Geometry check sheet. Reference: the model listing, model coordinates, mm. A direction names the side the tool comes from. Give positions to 0.01 mm unless a question says otherwise; leave off trailing zeros. Order: outer loops, then holes, each group sorted by start corner. A loop starts at its lowest first (then second) coordinate and runs counter-clockwise, first axis right, second up. Notation, with made-up numbers: M 77,68 L 96,68 A21 ccw 96,97 Z; hole C 79.5,-36 d7. An arc over 180 degrees is marked long. Use CSV: the item, a comma, the result in double quotes. Start each with the question number.
from build123d import *

# Parameters (mm, degrees)
SKETCH1_R                        = 8
BOSS_EXTRUDE1_DEPTH              = 21.88
BOSS_EXTRUDE2_DEPTH              = 26.5
SKETCH3_R                        = 2.835
BOSS_EXTRUDE3_DEPTH              = 2
BOSS_EXTRUDE4_DEPTH              = 10
F_2_05_2_05_DIAMETER_HOLE1_D     = 2.05
F_2_05_2_05_DIAMETER_HOLE1_DEPTH = 3
F_2_05_2_05_DIAMETER_HOLE1_TIP   = 0.615882135


with BuildPart() as part:
    # Sketch1 → Boss-Extrude1 (new body)
    with BuildSketch(Plane.XY):
        Circle(SKETCH1_R)
    extrude(amount=BOSS_EXTRUDE1_DEPTH)

    # Sketch2 → Boss-Extrude2 (add)
    with BuildSketch(Plane.XY.offset(21.88)):
        with BuildLine():
            Line((5.634523633, 5.0703593), (6.054375133, -4.560804945))
            ThreePointArc((6.054375133, -4.560804945), (0.33012154, -7.572807918), (-5.634523633, -5.0703593))
            Line((-5.634523633, -5.0703593), (-6.054375133, 4.560804945))
            ThreePointArc((-6.054375133, 4.560804945), (-0.33012154, 7.572807918), (5.634523633, 5.0703593))
        make_face()
    extrude(amount=BOSS_EXTRUDE2_DEPTH)

    # Sketch3 → Boss-Extrude3 (add)
    with BuildSketch(Plane(origin=(0, 0, 0), x_dir=(-1, 0, 0), z_dir=(0, 0, -1))):
        with Locations(Location((0, 0, 0), (0, 0, 180))):
            Circle(SKETCH3_R)
    extrude(amount=BOSS_EXTRUDE3_DEPTH)

    # Sketch4 → Boss-Extrude4 (add)
    with BuildSketch(Plane(origin=(0, 0, -2), x_dir=(-1, 0, 0), z_dir=(0, 0, -1))):
        with BuildLine():
            Line((0, 1.4), (-1.313042891, -0.485714286))
            ThreePointArc((-1.313042891, -0.485714286), (1.148912529, -0.8), (0, 1.4))
        make_face()
    extrude(amount=BOSS_EXTRUDE4_DEPTH)

    # Ø2.05 (2.05) Diameter Hole1
    with Locations(Plane(origin=(0, 0, 0), x_dir=(-1, 0, 0), z_dir=(0, 0, -1))):
        with Locations((-5.5, 0), (5.5, 0)):
            Hole(F_2_05_2_05_DIAMETER_HOLE1_D / 2, depth=F_2_05_2_05_DIAMETER_HOLE1_DEPTH)
            with Locations((0, 0, -(F_2_05_2_05_DIAMETER_HOLE1_DEPTH + F_2_05_2_05_DIAMETER_HOLE1_TIP / 2))):  # 118° drill point
                Cone(0, F_2_05_2_05_DIAMETER_HOLE1_D / 2, F_2_05_2_05_DIAMETER_HOLE1_TIP, mode=Mode.SUBTRACT)


solid = part.part
(1) Sectioned sample at B-B on z = 29.5. Record the cut outline in (x, y).
(2) Sectioned sample at A-A on y = -3.5. Record the cut outline in (x, z), then the cut area to 3 significant figures.
(3) Draft check along Y on faces 4 (the face through (0, 0, -12)), 5 (the face through (5.84, 0.32, 34.94)), 6 (the face through (-5.66, -0.07, 3.51)), 7 (the face through (-6.524, 0.045, 1.521)). Enter one of: +Y half, -Y half, draft (parallel to the pull), parting line (faces both ways), or undercut.
(4) Sectioned sample at D-D on z = 19. Record the cut outline in (x, y), then the cut area to 3 significant figures.
(5) Sectioned sample at C-C on x = 2. Record the cut outline in (y, z).
(6) Go/stop test with flat-tipped pins: P1, Ø1.5, axis at y = 2.5, z = 10.5, coming from the -X side; P2, Ø3, axis at y = 6, z = 1.5, coming from the +X side; P3, Ø1, axis at x = -3, z = 42, coming from the +Y side. Record where each tip stops, or that it passes through.
(7) Access from +Z, -Z, +X, -X, +Y, -Y to the whole of each face (thin tool, end or side, straight path). Record for faces 1 (the face through (0.65, 0.47, -6.93)), 2 (the face through (1, 1, -2)), 3 (the face through (-5.84, -0.32, 34.94)).
(8) Thickness scan on line 1 (Z direction, x = 4.5, y = 1.25); line 2 (Z direction, x = -6.5, y = 3); line 3 (Y direction, x = -5.5, z = 2.35) (3 decimals). Record the ranges inside material, lowest first.
Responses:
1,outline,"M -6.05,4.56 L -5.63,-5.07 A7.58 ccw 6.05,-4.56 L 5.63,5.07 A7.58 ccw Z"
2,outline,"M -7.19,0 L 7.19,0 L 7.19,21.88 L 6.01,21.88 L 6.01,48.38 L -5.7,48.38 L -5.7,21.88 L -7.19,21.88 Z"
2,area,"625 mm2"
3,face 4,"draft"
3,face 5,"+Y half"
3,face 6,"undercut"
3,face 7,"undercut"
4,outline,"C 0,0 d16"
4,area,"201 mm2"
5,outline,"M -7.75,0 L -2.01,0 L -2.01,-2 L 2.01,-2 L 2.01,0 L 7.75,0 L 7.75,21.88 L 7.31,21.88 L 7.31,48.38 L -7.31,48.38 L -7.31,21.88 L -7.75,21.88 Z"
6,P1,"x = -7.81"
6,P2,"x = 6.61"
6,P3,"y = 7.16"
7,face 1,"-Z, +X, +Y"
7,face 2,"-Z"
7,face 3,"+Z, -X, -Y"
8,line 1,"0 to 48.38"
8,line 2,"0 to 21.88"
8,line 3,"-5.809 to -1.025, 1.025 to 5.809"
